```python
from build123d import *

# Parameters (mm, degrees)
SKETCH1_R           = 250
BOSS_EXTRUDE1_DEPTH = 20
SKETCH2_R           = 12.5
CUT_EXTRUDE1_DEPTH  = 20


with BuildPart() as part:
    # Sketch1 → Boss-Extrude1 (new body)
    with BuildSketch(Plane(origin=(0, 0, 0), x_dir=(1, 0, 0), z_dir=(0, 1, 0))):
        with Locations(Location((0, 0, 0), (0, 0, 270))):
            Circle(SKETCH1_R)
    extrude(amount=BOSS_EXTRUDE1_DEPTH)

    # Sketch2 → Cut-Extrude1 (cut)
    with BuildSketch(Plane(origin=(0, 20, 0), x_dir=(1, 0, 0), z_dir=(0, 1, 0))):
        with Locations(Location((0, 217.5, 0), (0, 0, 270))):
            Circle(SKETCH2_R)
        with Locations(Location((108.75, 188.360525323, 0), (0, 0, 270))):
            Circle(SKETCH2_R)
        with Locations(Location((188.360525323, 108.75, 0), (0, 0, 270))):
            Circle(SKETCH2_R)
        with Locations(Location((217.5, 0, 0), (0, 0, 270))):
            Circle(SKETCH2_R)
        with Locations(Location((188.360525323, -108.75, 0), (0, 0, 270))):
            Circle(SKETCH2_R)
        with Locations(Location((108.75, -188.360525323, 0), (0, 0, 270))):
            Circle(SKETCH2_R)
        with Locations(Location((0, -217.5, 0), (0, 0, 270))):
            Circle(SKETCH2_R)
        with Locations(Location((-108.75, -188.360525323, 0), (0, 0, 270))):
            Circle(SKETCH2_R)
        with Locations(Location((-188.360525323, -108.75, 0), (0, 0, 270))):
            Circle(SKETCH2_R)
        with Locations(Location((-217.5, 0, 0), (0, 0, 270))):
            Circle(SKETCH2_R)
        with Locations(Location((-188.360525323, 108.75, 0), (0, 0, 270))):
            Circle(SKETCH2_R)
        with Locations(Location((-108.75, 188.360525323, 0), (0, 0, 270))):
            Circle(SKETCH2_R)
    extrude(amount=-CUT_EXTRUDE1_DEPTH, mode=Mode.SUBTRACT)


solid = part.part
```
Part model, mm, in its own coordinate system. Give positions to 0.01 mm unless a question says otherwise; leave off trailing zeros. Order: outer loops, then holes, each group sorted by start corner. A loop starts at its lowest first (then second) coordinate and runs counter-clockwise, first axis right, second up. Notation, with made-up numbers: M -15,-2.5 L 33,-2.5 A8 ccw 33,6.5 Z; hole C -30.5,-4.75 d3. An arc over 180 degrees is marked long. Use a Markdown table: item, result. Add a question column.
(1) Saw through at B-B, the plane x = 108.75. Give the cut face in (y, z), and give its area (3 significant figures).
(2) Mould opens along X. For faces 1 (the face through (121.144, 10.14, -189.988)), 2 (the face through (10.99, 9.86, -249.76)), 3 (the face through (4, 20, -3)), 4 (the face through (-4.788, 10.14, -205.953)) say: +X half, -X half, draft (parallel to the pull), parting line (faces both ways), or undercut.
(3) Saw through at A-A, the plane z = 0. Give the cut face in (x, y), and give its area (3 significant figures).
(4) Probe line 1 along X through (y, z) = (1.5, 11.5); line 2 along X through (y, z) = (15.25, 0); line 3 along Z through (x, y) = (-10, 1.75). List the from-to ranges inside material, lowest first. Write a range as [from, to].
(5) Drop flat-ended pins along their axis: P1, Ø20, axis at x = 0, z = -217.5, coming from the -Y side; P2, Ø2, axis at y = 5.5, z = 116.5, coming from the -X side; P3, Ø1.5, axis at x = -60, y = 16, coming from the +Z side; P4, Ø3, axis at x = 57.5, y = 9.5, coming from the +Z side. Give the stop position or say it passes through.
(6) Saw through at C-C, the plane z = 217.5. Give the cut face in (x, y), and give its area (3 significant figures).
(7) Saw through at D-D, the plane x = -217.5. Give the cut face in (y, z).
Answer key:
| question | item | result |
|---|---|---|
| 1 | outline | M 0,-225.11 L 20,-225.11 L 20,-200.86 L 0,-200.86 Z; M 0,-175.86 L 20,-175.86 L 20,175.86 L 0,175.86 Z; M 0,200.86 L 20,200.86 L 20,225.11 L 0,225.11 Z |
| 1 | area | 8,000 mm^2 |
| 2 | face 1 | undercut |
| 2 | face 2 | parting line |
| 2 | face 3 | draft |
| 2 | face 4 | undercut |
| 3 | outline | M -250,0 L -230,0 L -230,20 L -250,20 Z; M -205,0 L 205,0 L 205,20 L -205,20 Z; M 230,0 L 250,0 L 250,20 L 230,20 Z |
| 3 | area | 9,000 mm^2 |
| 4 | line 1 | [-249.74, -222.4], [-212.6, 212.6], [222.4, 249.74] |
| 4 | line 2 | [-250, -230], [-205, 205], [230, 250] |
| 4 | line 3 | [-249.8, -225], [-210, 210], [225, 249.8] |
| 5 | P1 | through |
| 5 | P2 | x = -221.72 |
| 5 | P3 | z = 242.88 |
| 5 | P4 | z = 243.65 |
| 6 | outline | M -123.26,0 L -12.5,0 L -12.5,20 L -123.26,20 Z; M 12.5,0 L 123.26,0 L 123.26,20 L 12.5,20 Z |
| 6 | area | 4,430 mm^2 |
| 7 | outline | M 0,-123.26 L 20,-123.26 L 20,-12.5 L 0,-12.5 Z; M 0,12.5 L 20,12.5 L 20,123.26 L 0,123.26 Z |
